from build123d import *

# Parameters (mm, degrees)
F1_DEPTH = 4
F2_R     = 0.5
F3_R     = 1
F4_R     = 1
F5_R     = 1.5
F6_DEPTH = 25.4


# Not quite as in the source:
# - a feature names something its author has since deleted; it is built from what else it names


with BuildPart() as f1:
    # F0 (on Top) → F1 (new body)
    with BuildSketch(Plane.XY):
        with BuildLine():
            ThreePointArc((-2.1499598203, -14.279765827), (-8.9479939511, 2.1344933303), (0, 17.482932208))
            Line((0, 17.482932208), (0, 40))
            ThreePointArc((0, 40), (-17.5115843593, 34.3056723382), (-25, 17.482932208))
            ThreePointArc((-25, 17.482932208), (-17.8797085459, 27.1675710157), (-6.0147373006, 29.0945470333))
            Line((-6.0147373006, 29.0945470333), (-6.0147373006, 19.0945470333))
            ThreePointArc((-6.0147373006, 19.0945470333), (-13.7044570112, 4.575418106), (-10.7216048739, -11.5812983662))
            ThreePointArc((-10.7216048739, -11.5812983662), (-10.6011415068, -11.9319286193), (-10.6166990692, -12.3023485965))
            Line((-10.6166990692, -12.3023485965), (-16.3921895572, -37.1448185197))
            ThreePointArc((-16.3921895572, -37.1448185197), (-11.0096096716, -45.0763845561), (-3.5247629898, -39.0881480742))
            Line((-3.5247629898, -39.0881480742), (-1.8103202737, -15.1042462433))
            ThreePointArc((-1.8103202737, -15.1042462433), (-1.8831553034, -14.6520537771), (-2.1499598203, -14.279765827))
        make_face()
    extrude(amount=-F1_DEPTH)

    # F2
    f2_edges = [f1.edges().sort_by_distance(p)[0] for p in [
        (-25, 17.482932, -2),
    ]]
    fillet(f2_edges, radius=F2_R)

    # F3
    f3_edges = [f1.edges().sort_by_distance(p)[0] for p in [
        (-6.014737, 24.094547, 0),
        (-6.014737, 24.094547, -4),
        (-13.704457, 4.575418, 0),
    ]]
    fillet(f3_edges, radius=F3_R)

    # F4
    f4_edges = [f1.edges().sort_by_distance(p)[0] for p in [
        (-13.704457, 4.575418, -4),
    ]]
    fillet(f4_edges, radius=F4_R)

    # F5 (on face) → F6 (cut)
    with BuildSketch(Plane.XY):
        with Locations((-5, -15.8231072128)):
            Circle(F5_R)
        with Locations((-10.0349408695, -38.6227806321)):
            Circle(F5_R)
    extrude(amount=-F6_DEPTH, mode=Mode.SUBTRACT)


solid = f1.part
Part model, mm, in its own coordinate system. A direction names the side the tool comes from. Coordinates: 2 decimals unless noted, no trailing zeros. Loops run counter-clockwise (first coordinate to the right, second up) from the corner with the lowest first, then second, coordinate; pieces in that order, holes last. Notation, with made-up numbers: M 29,-20.75 L 82,-20.75 A19 cw 82,13.25 Z; hole C 39.25,23 d7. An arc over 180 degrees is marked long. Use a Markdown table: item, result. Add a question column.
Q1. Which spindle directions (+Z, -Z, +X, -X, +Y, -Y) get a long thin tool onto all of the face, cutting with end or side? Do faces 1 (the flat face through (-6.015, 24, -2)), 2 (the flat face through (-13.464, -24.55, -1.986)), 3 (the cylindrical face through (-13.171, -24.618, -3.715)). Say none if no direction does.
Q2. Probe L1, parallel to Y at x = -5, z = -2.1; L2, parallel to Y at x = -5.25, z = -3.3; L3, parallel to X at y = 27.5, z = -1.55. List the from-to ranges inside material, lowest first.
Q3. Cut at A-A (y = 25.5). Write the cut outline in (x, z), and give its area (3 significant figures).
Q4. Pin check, flat tips, straight feed: P1, Ø2, axis at y = 9.5, z = -2.5, coming from the +X side; P2, Ø2, axis at y = 24.5, z = -2, coming from the -X side. Stop position of each tip, or through.
Q5. Mould opens along Y. For faces 4 (the flat face through (0, 29, -2)), 5 (the cylindrical face through (-15.931, 35.605, -1.972)), 6 (the cylindrical face through (-13.252, -24.966, -0.285)), 7 (the cylindrical face through (-2.955, -26.907, -0.285)) say: +Y half, -Y half, draft (parallel to the pull), parting line (faces both ways), or undercut.
Q6. Cut at B-B (z = -2.15). Give the number of separate pieces and of enclosed holes in the cut face, and give its area (3 significant figures).
Worked out:
| question | item | result |
|---|---|---|
| 1 | face 1 | +Z, -Z |
| 1 | face 2 | +Z, -Z, -X |
| 1 | face 3 | -Z, -X |
| 2 | L1 | y = -42.78 to -17.32, -14.32 to -11.21, 12.78 to 39.97 |
| 2 | L2 | y = -42.99 to -17.3, -14.34 to -10.95, 12.51 to 39.94 |
| 2 | L3 | x = -22.66 to -17.31, -6.01 to 0 |
| 3 | outline | M -23.53,-4 L -20.13,-4 L -20.13,0 L -23.53,0 Z; M -6.01,-3 A1 ccw -5.01,-4 L 0,-4 L 0,0 L -5.01,0 A1 ccw -6.01,-1 Z |
| 3 | area | 37.2 mm2 |
| 4 | P1 | stops at x = -6.47 |
| 4 | P2 | stops at x = -24.19 |
| 5 | face 4 | draft |
| 5 | face 5 | +Y half |
| 5 | face 6 | undercut |
| 5 | face 7 | -Y half |
| 6 | separate pieces | 1 |
| 6 | enclosed holes | 2 |
| 6 | area | 783 mm2 |
